Here's how the part is built. I have some questions about the finished solid (model axes, mm). Face numbers are marked on the shaded views. A direction names the side the tool comes from. Round coordinates to 2 decimals unless told otherwise and drop trailing zeros. Loops run counter-clockwise (first coordinate to the right, second up) from the corner with the lowest first, then second, coordinate; pieces in that order, holes last. Notation, with made-up numbers: (86, 33) -> (124, 33) arc R22 cw to (124, 44) -> close; hole circle Ø11 at (11.25, -4.75). An arc over 180 degrees is marked (long way). Use one line per item in the form item = value. Start each with the question number.
Item 1: If we section it at C-C (x = 2.5): Write out the boundary of the cut face in (y, z).
Item 2: I'm going to push flat-ended pins straight in: pin 1 Ø1.5 at (y, z) = (-1.5, -1) entering from -X; pin 2 Ø7 at (x, y) = (-0.5, 0) entering from +Z; pin 3 Ø1 at (x, y) = (-5, 21.5) entering from +Z. Where does each tip first touch, or does it pass through?
Item 3: If we section it at D-D (z = -3.25): State how many separate pieces and enclosed holes the cut face has, then the cut area to 3 significant figures.
Item 4: For the marked faces 4, 5 and 6, which set-ups out of +Z, -Z, +X, -X, +Y, -Y let a thin tool reach every point of the face, with its end or its side?
Item 5: If I drill on L1, parallel to X at y = 14.5, z = 0.5; L2, parallel to Z at x = 4, y = 1.75; L3, parallel to Y at x = 1.75, z = 0.5, over which ranges is the centre line in solid material (lowest first)? Write a range as [from, to].
Item 6: Thinking about a two-plate mould opening in X: for the marked faces 1, 2 and 3, which applies, released by +X, released by -X, zero draft, split by the parting line, or undercut?
Item 7: If we section it at A-A (y = 0): Write out the boundary of the cut face in (x, z).
Item 8: If we section it at B-B (x = 0): Write out the boundary of the cut face in (y, z).
```python
from build123d import *

# Parameters (mm, degrees)
SKETCH1_W               = 10
SKETCH1_H               = 10
BOSS_EXTRUDE1_DEPTH     = 3.75
SKETCH2_W               = 6.5
SKETCH2_H               = 6.5
CUT_EXTRUDE1_DEPTH      = 5
BOSS_EXTRUDE2_DEPTH     = 7.5
M2_CLEARANCE_HOLE1_D    = 2.4
FILLET5_R               = 1
FILLET1_R               = 1
FILLET3_R               = 1
SKETCH17_R              = 5
CUT_EXTRUDE2_DEPTH      = 7
SKETCH5_R               = 1.5875
CUT_EXTRUDE3_DEPTH      = 5
FILLET4_R               = 1
CUT_EXTRUDE4_REACH      = 34.182
CUT_EXTRUDE4_END_RADIUS = 5
SKETCH18_R              = 1.35


with BuildPart() as part:
    # Sketch1 → Boss-Extrude1 (new, symmetric)
    with BuildSketch(Plane.XY):
        Rectangle(SKETCH1_W, SKETCH1_H)
    extrude(amount=BOSS_EXTRUDE1_DEPTH, both=True)

    # Sketch2 → Cut-Extrude1 (cut)
    with BuildSketch(Plane(origin=(0, 0, -3.75), x_dir=(-1, 0, 0), z_dir=(0, 0, -1))):
        Rectangle(SKETCH2_W, SKETCH2_H)
    extrude(amount=-CUT_EXTRUDE1_DEPTH, mode=Mode.SUBTRACT)

    # Sketch3 → Boss-Extrude2 (add, symmetric)
    with BuildSketch(Plane(origin=(0, 0, 0), x_dir=(0, 0, -1), z_dir=(1, 0, 0))):
        Polygon((-6.25, 5), (5, 24.485571585), (12.5, 20.155444566), (3.75, 5), align=None)
    extrude(amount=BOSS_EXTRUDE2_DEPTH, both=True)

    # M2 Clearance Hole1 (through all)
    with Locations(Plane.XY.offset(3.75)):
        with Locations((0, 0)):
            Hole(M2_CLEARANCE_HOLE1_D / 2)

    # Fillet5
    fillet5_edges = [part.edges().sort_by_distance(p)[0] for p in [
        (-7.5, 5, 1.25),
        (-7.5, 22.320508076, -8.75),
        (7.5, 5, 1.25),
        (7.5, 22.320508076, -8.75),
    ]]
    fillet(fillet5_edges, radius=FILLET5_R)

    # Fillet1
    fillet1_edges = [part.edges().sort_by_distance(p)[0] for p in [
        (-5, 5, 0),
        (5, 5, 0),
    ]]
    fillet(fillet1_edges, radius=FILLET1_R)

    # Fillet3
    fillet3_edges = [part.edges().sort_by_distance(p)[0] for p in [
        (5, -5, 0),
        (-5, -5, 0),
    ]]
    fillet(fillet3_edges, radius=FILLET3_R)

    # Sketch17 → Cut-Extrude2 (cut)
    with BuildSketch(Plane(origin=(0, 3.956329387, 6.852563509), x_dir=(1, 0, 0), z_dir=(0, 0.5000000000000039, 0.8660254037844365))):
        with Locations(Location((0, 13.705127019, 0), (0, 0, 270))):
            Circle(SKETCH17_R)
    extrude(amount=-CUT_EXTRUDE2_DEPTH, mode=Mode.SUBTRACT)

    # Sketch5 → Cut-Extrude3 (cut)
    with BuildSketch(Plane(origin=(0, -0.373797632, -0.647436491), x_dir=(-1, 0, 0), z_dir=(0, -0.5000000000000038, -0.8660254037844366))):
        with Locations(Location((0, 13.705127019, 0), (0, 0, 90))):
            Circle(SKETCH5_R)
    extrude(amount=-CUT_EXTRUDE3_DEPTH, mode=Mode.SUBTRACT)

    # Fillet4
    fillet4_edges = [part.edges().sort_by_distance(p)[0] for p in [
        (0, 5, 3.75),
    ]]
    fillet(fillet4_edges, radius=FILLET4_R)

    # Cut-Extrude4: up to this cylinder (the profile starts outside it)
    cut_extrude4_end = Plane(origin=(0, 14.075317613, -3.031088799), z_dir=(0, 0.5000000000000039, 0.8660254037844365)) * Cylinder(CUT_EXTRUDE4_END_RADIUS, 79.364, mode=Mode.PRIVATE)
    # Sketch18 → Cut-Extrude4 (cut, up to the surface)
    with BuildSketch(Plane(origin=(0, 20.529242198, -11.852563509), x_dir=(1, 0, 0), z_dir=(0, 0.8660254037844366, -0.5000000000000038)), mode=Mode.PRIVATE) as cut_extrude4_sk1:
        with Locations(Location((0, -4.412658774, 0), (0, 0, 270))):
            Circle(SKETCH18_R)
    cut_extrude4_tool1 = extrude(cut_extrude4_sk1.sketch, amount=-CUT_EXTRUDE4_REACH, mode=Mode.PRIVATE) - cut_extrude4_end
    add(cut_extrude4_tool1.solids().sort_by_distance((0, 22.735572, -8.031089))[0], mode=Mode.SUBTRACT)


solid = part.part
```
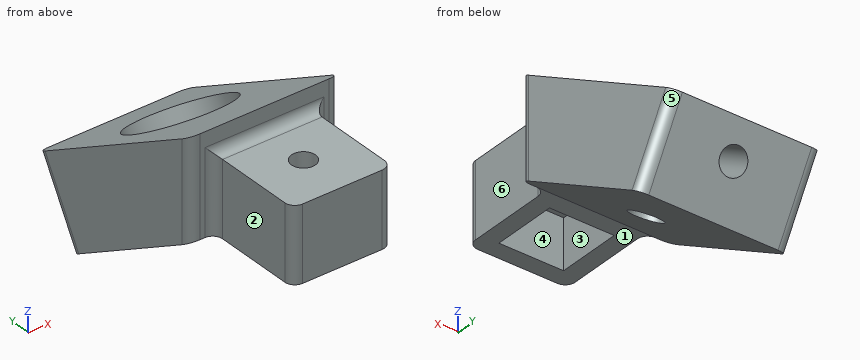
Values found:
q1.outline = (-5, -3.75) -> (-3.25, -3.75) -> (-3.25, 1.25) -> (3.25, 1.25) -> (3.25, -3.75) -> (5, -3.75) -> (20.16, -12.5) -> (24.49, -5) -> (19.58, -2.17) -> (16.08, -8.23) -> (8.58, -3.9) -> (12.08, 2.17) -> (5, 6.25) -> (5, 4.75) arc R1 cw to (4, 3.75) -> (-5, 3.75) -> close
q2.pin_1 = -5
q2.pin_2 = 3.75
q2.pin_3 = -2.99
q3.separate_pieces = 1
q3.enclosed_holes = 2
q3.area = 213 mm2
q4.face_4 = -Z
q4.face_5 = -Z, +X, +Y
q4.face_6 = +Z, -Z, +X, -Y
q5.L1 = [-7.5, -4.8], [4.8, 7.5]
q5.L2 = [-3.75, 3.75]
q5.L3 = [-5, -3.25], [3.25, 10.71]
q6.face_1 = zero draft
q6.face_2 = released by -X
q6.face_3 = undercut
q7.outline = (-5, -3.75) -> (-3.25, -3.75) -> (-3.25, 1.25) -> (-1.2, 1.25) -> (-1.2, 3.75) -> (-5, 3.75) -> close; (1.2, 1.25) -> (3.25, 1.25) -> (3.25, -3.75) -> (5, -3.75) -> (5, 3.75) -> (1.2, 3.75) -> close
q8.outline = (-5, -3.75) -> (-3.25, -3.75) -> (-3.25, 1.25) -> (-1.2, 1.25) -> (-1.2, 3.75) -> (-5, 3.75) -> close; (1.2, 1.25) -> (3.25, 1.25) -> (3.25, -3.75) -> (5, -3.75) -> (10.12, -6.71) -> (10.95, -5.27) -> (8, -3.56) -> (11.5, 2.5) -> (5, 6.25) -> (5, 4.75) arc R1 cw to (4, 3.75) -> (1.2, 3.75) -> close; (12.87, -8.29) -> (20.16, -12.5) -> (22.06, -9.2) -> (17.73, -6.7) -> (16.66, -8.56) -> (13.7, -6.86) -> close; (19.08, -4.36) -> (23.41, -6.86) -> (24.49, -5) -> (20.16, -2.5) -> close
